Design review of the part built by this model. Coordinates are the model's own, in mm. A direction names the side the tool comes from. Round coordinates to 2 decimals unless told otherwise and drop trailing zeros. Use one line per item in the form item = value.
```python
from build123d import *

# Parameters (mm, degrees)
F1_R          = 1.45
F6_DEPTH      = 0.201
F6_DEPTH_BACK = 3.001
F7_R          = 1
F8_SIZE       = 0.19999


# Not quite as in the source:
# - a fillet or chamfer is up to 0.001 mm smaller than in the source, because OpenCascade refuses the exact size


with BuildPart() as f4:
    # F4: sweep along a path in F2
    with BuildLine(Plane.XZ) as f4_path:
        Line((0, 0), (0, -0.2))
    # F3 (on Top) → F4 (sweep)
    with BuildSketch(Plane.XY):
        Polygon((16.5, 16.5), (0, 16.5), (-16.5, 16.5), (-16.5, 0), (-16.5, -16.5), (0, -16.5), (16.5, -16.5), (16.5, 0), align=None)
        Polygon((0, 13.5), (8, 13.5), (13.5, 13.5), (13.5, 8), (13.5, 0), (13.5, -8), (13.5, -13.5), (8, -13.5), (0, -13.5), (-8, -13.5), (-13.5, -13.5), (-13.5, -8), (-13.5, 0), (-13.5, 8), (-13.5, 13.5), (-8, 13.5), align=None, mode=Mode.SUBTRACT)
        Polygon((-10, -8), (-13.5, -8), (-13.5, -13.5), (-8, -13.5), (-8, -10), (-10, -10), align=None)
        Polygon((-8, 10), (-8, 13.5), (-13.5, 13.5), (-13.5, 8), (-10, 8), (-10, 10), align=None)
        Polygon((8, 13.5), (8, 10), (10, 10), (10, 8), (13.5, 8), (13.5, 13.5), align=None)
        Polygon((13.5, -13.5), (13.5, -8), (10, -8), (10, -10), (8, -10), (8, -13.5), align=None)
    sweep(path=f4_path.line)

    # F5: sweep along a path in F2
    with BuildLine(Plane.XZ) as f5_path:
        Line((0, 0), (0, 3))
    # F3 (on Top) → F5 (sweep)
    with BuildSketch(Plane.XY):
        Polygon((-8, 10), (-8, 13.5), (-13.5, 13.5), (-13.5, 8), (-10, 8), (-10, 10), align=None)
        Polygon((8, 13.5), (8, 10), (10, 10), (10, 8), (13.5, 8), (13.5, 13.5), align=None)
        Polygon((-10, -8), (-13.5, -8), (-13.5, -13.5), (-8, -13.5), (-8, -10), (-10, -10), align=None)
        Polygon((13.5, -13.5), (13.5, -8), (10, -8), (10, -10), (8, -10), (8, -13.5), align=None)
    sweep(path=f5_path.line)

    # F1 (on Top) → F6 (cut, two sides)
    with BuildSketch(Plane.XY) as f6_sk:
        with Locations((10, 10)):
            Circle(F1_R)
        with Locations((-10, 10)):
            Circle(F1_R)
        with Locations((-10, -10)):
            Circle(F1_R)
        with Locations((10, -10)):
            Circle(F1_R)
    extrude(amount=-F6_DEPTH, mode=Mode.SUBTRACT)
    extrude(f6_sk.sketch, amount=F6_DEPTH_BACK, mode=Mode.SUBTRACT)

    # F7
    f7_edges = [f4.edges().sort_by_distance(p)[0] for p in [
        (16.5, 16.5, -0.1),
        (13.5, -13.5, 1.5),
        (13.5, 13.5, 1.5),
        (-13.5, -13.5, 1.5),
        (-16.5, -16.5, -0.1),
        (-13.5, 13.5, 1.5),
        (-16.5, 16.5, -0.1),
    ]]
    fillet(f7_edges, radius=F7_R)

    # F8 (size 0.2 in the source; OpenCascade refuses exactly that, so slightly less here)
    f8_edges = [f4.edges().sort_by_distance(p)[0] for p in [
        (0, 16.5, -0.2),
        (16.207107, 16.207107, -0.2),
        (-16.207107, 16.207107, -0.2),
        (16.5, -0.5, -0.2),
        (-16.5, 0, -0.2),
        (0.5, -16.5, -0.2),
        (-16.207107, -16.207107, -0.2),
        (-13.5, 0, -0.2),
        (-11.75, 8, -0.2),
        (-10, 8.275, -0.2),
        (-11.025305, 11.025305, -0.2),
        (-8.275, 10, -0.2),
        (-8, 11.75, -0.2),
        (0, 13.5, -0.2),
        (8, 11.75, -0.2),
        (8.275, 10, -0.2),
        (11.025305, 11.025305, -0.2),
        (10, 8.275, -0.2),
        (11.75, 8, -0.2),
        (13.5, 0, -0.2),
        (11.75, -8, -0.2),
        (10, -8.275, -0.2),
        (11.025305, -11.025305, -0.2),
        (8.275, -10, -0.2),
        (8, -11.75, -0.2),
        (0, -13.5, -0.2),
        (-8, -11.75, -0.2),
        (-8.275, -10, -0.2),
        (-11.025305, -11.025305, -0.2),
        (-10, -8.275, -0.2),
        (-11.75, -8, -0.2),
    ]]
    chamfer(f8_edges, length=F8_SIZE)


solid = f4.part
```
Q1. Draft analysis for pull direction X (two halves, no side actions). For faces 1 (the flat face through (8, -12, 1)), 2 (the flat face through (11.3, 11.4, 3)), 3 (the cylindrical face through (-13.199, 13.215, 1.521)), state which applies: released by +X, released by -X, zero draft, split by the parting line, or undercut.
Calculated:
face_1 = undercut
face_2 = zero draft
face_3 = released by -X
Q2. Machinability: for faces 4 (the flat face through (-8, -12, 1)), 5 (the flat face through (12, -8, 1)), 6 (the flat face through (-10, 13.5, 2)), 7 (the flat face through (-10, -13.5, 2)), 8 (the cylindrical face through (13.215, -13.199, 1.521)), which of the approach directions +Z, -Z, +X, -X, +Y, -Y give a long, thin tool a straight path to every point of the face, cutting with its end or side? Answer none if there is none.
Calculated:
face_4 = +Z, -Z, +Y, -Y
face_5 = +Z, -Z, +X, -X
face_6 = +Z, +X, -X, +Y
face_7 = +Z, +X, -X, -Y
face_8 = +Z, +X, -Y
Q3. For P1, Ø1.5, axis at y = -12, z = 1.5, coming from the +X side; P2, Ø1, axis at x = 10.5, z = 1.5, coming from the -Y side, all flat-tipped, find the tip position at first contact; note any pin that passes through.
Calculated:
P1 = 13.5
P2 = -13.5
Q4. To check wall thickness, follow line 1 along Y through (x, z) = (-10.5, 2.55); line 2 along Y through (x, z) = (11.5, 2.1). State the ranges of each line that lie inside material, in increasing order. Write a range as from..to.
Calculated:
line_1 = -13.5..-11.36, -8.64..-8, 8..8.64, 11.36..13.5
line_2 = -13.5..-8, 8..13.5
Q5. We need section B-B on z = 2.15. State how many separate pieces and enclosed holes the cut face has, then the cut area to 3 significant figures.
Calculated:
separate_pieces = 4
enclosed_holes = 0
area = 84.3 mm2
